For this review, take the finished solid that the model builds, in its own axes (mm). A direction names the side the tool comes from. Give positions to 0.01 mm unless a question says otherwise; leave off trailing zeros. Loops run counter-clockwise (first coordinate to the right, second up) from the corner with the lowest first, then second, coordinate; pieces in that order, holes last. Notation, with made-up numbers: (-22, 38) - (-13, 38) arc R31 ccw to (-13, 67) - close; hole circle Ø2 at (59.5, 32). An arc over 180 degrees is marked (long way). Answer in a Markdown table with one row per item.
```python
from build123d import *

# Parameters (mm, degrees)
F0_W     = 18
F0_H     = 18
F0_R     = 7
F1_DEPTH = 45
F0_R_2   = 3.75
F2_DEPTH = 25
F3_R     = 2
F4_DEPTH = 25
F5_R     = 1


with BuildPart() as f1:
    # F0 (on Front) → F1 (new body)
    with BuildSketch(Plane.XZ):
        with Locations((-0.41628, 1.888414)):
            Rectangle(F0_W, F0_H)
        with Locations((-0.41628, 1.888414)):
            Circle(F0_R, mode=Mode.SUBTRACT)
    extrude(amount=F1_DEPTH)

    # F0 (on Front) → F2 (join)
    with BuildSketch(Plane.XZ):
        with Locations((-0.41628, 1.888414)):
            Circle(F0_R)
        with Locations((-0.41628, 1.888414)):
            Circle(F0_R_2, mode=Mode.SUBTRACT)
    extrude(amount=F2_DEPTH)

    # F3 (on face) → F4 (cut)
    with BuildSketch(Plane(origin=(0, 0, -7.111586), x_dir=(1, 0, 0), z_dir=(0, 0, -1))):
        with Locations((0, 22)):
            Circle(F3_R)
    extrude(amount=-F4_DEPTH, mode=Mode.SUBTRACT)

    # F5
    f5_edges = [f1.edges().sort_by_distance(p)[0] for p in [
        (-9.41628, -22.5, -7.111586),
        (8.58372, -22.5, -7.111586),
        (-9.41628, -22.5, 10.888414),
        (8.58372, -22.5, 10.888414),
        (-9.41628, 0, 1.888414),
        (-0.41628, 0, 10.888414),
        (-0.41628, 0, -7.111586),
        (8.58372, 0, 1.888414),
        (8.58372, -45, 1.888414),
        (-0.41628, -45, 10.888414),
        (-9.41628, -45, 1.888414),
        (-0.41628, -45, -7.111586),
    ]]
    fillet(f5_edges, radius=F5_R)


solid = f1.part
```
1. We need section C-C, the plane y = -21. Give the boundary of the cut face in (x, z).
Values:
| item | result |
|---|---|
| outline | (-9.42, -6.11) arc R1 ccw to (-8.42, -7.11) - (-1.73, -7.11) - (-1.73, -1.62) arc R3.75 cw to (-1.73, 5.4) - (-1.73, 10.89) - (-8.42, 10.89) arc R1 ccw to (-9.42, 9.89) - close; (1.73, -7.11) - (7.58, -7.11) arc R1 ccw to (8.58, -6.11) - (8.58, 9.89) arc R1 ccw to (7.58, 10.89) - (1.73, 10.89) - (1.73, 4.96) arc R3.75 cw to (1.73, -1.19) - close |
2. For faces 5 (the face through (-8, -45, 2)), 6 (the face through (3, -25, -1)), list the 3-axis set-ups (+Z, -Z, +X, -X, +Y, -Y) from which the entire face can be reached by the end or side of a thin tool; tool diameter is ignored.
Values:
| item | result |
|---|---|
| face 5 | +Z, -Z, +X, -X, -Y |
| face 6 | -Y |
3. Mouldability with a two-part tool opening along X and no side actions: class faces 1 (the face through (-0.3, -0.3, 10.6)), 2 (the face through (1.908, -22.601, -4.088)), 3 (the face through (-9.13, -22.8, -6.81)), 4 (the face through (8.584, -22, 2)) as released by +X, released by -X, zero draft, split by the parting line, or undercut.
Values:
| item | result |
|---|---|
| face 1 | zero draft |
| face 2 | undercut |
| face 3 | released by -X |
| face 4 | released by +X |
4. We need section D-D, the plane y = -9.5. Give the boundary of the cut face in (x, z).
Values:
| item | result |
|---|---|
| outline | (-9.42, -6.11) arc R1 ccw to (-8.42, -7.11) - (7.58, -7.11) arc R1 ccw to (8.58, -6.11) - (8.58, 9.89) arc R1 ccw to (7.58, 10.89) - (-8.42, 10.89) arc R1 ccw to (-9.42, 9.89) - close; hole circle Ø7.5 at (-0.42, 1.89) |
5. Wall thickness on line 1 (X direction, y = -22, z = 7.75); line 2 (Y direction, x = 0, z = -3); line 3 (Y direction, x = -6, z = 10): over which ranges is each line inside the solid? List them lowest first. Write a range as [from, to].
Values:
| item | result |
|---|---|
| line 1 | x = [-9.42, -2], [2, 8.58] |
| line 2 | y = [-25, -24], [-20, 0] |
| line 3 | y = [-44.99, -0.01] |
6. Clearance check with a flat-ended pin moving along its axis: pin 1 (1 mm diameter, centred on x = -2, z = -4, fed in from -Y). State where the tip first meets the part, or that it passes through.
Values:
| item | result |
|---|---|
| pin 1 | stops at y = -25 |
7. We need section A-A, the plane x = 0. Give the boundary of the cut face in (y, z), and give its area (3 significant figures).
Values:
| item | result |
|---|---|
| outline | (-45, -6.11) arc R1 ccw to (-44, -7.11) - (-24, -7.11) - (-24, -1.84) - (-25, -1.84) - (-25, -5.1) - (-45, -5.1) - close; (-45, 8.88) - (-25, 8.88) - (-25, 5.62) - (-24, 5.62) - (-24, 10.89) - (-44, 10.89) arc R1 ccw to (-45, 9.89) - close; (-20, -7.11) - (-1, -7.11) arc R1 ccw to (0, -6.11) - (0, -1.84) - (-20, -1.84) - close; (-20, 5.62) - (0, 5.62) - (0, 9.89) arc R1 ccw to (-1, 10.89) - (-20, 10.89) - close |
| area | 301 mm^2 |
8. We need section B-B, the plane z = 1.25. Give the boundary of the cut face in (x, y), and give its area (3 significant figures).
Values:
| item | result |
|---|---|
| outline | (-9.42, -44) arc R1 ccw to (-8.42, -45) - (-7.39, -45) - (-7.39, -25) - (-4.11, -25) - (-4.11, 0) - (-8.42, 0) arc R1 ccw to (-9.42, -1) - close; (3.28, -25) - (6.55, -25) - (6.55, -45) - (7.58, -45) arc R1 ccw to (8.58, -44) - (8.58, -1) arc R1 ccw to (7.58, 0) - (3.28, 0) - close |
| area | 346 mm^2 |
